The listing builds one solid part. Answer for the finished solid, in the listing's coordinates (mm). Round coordinates to 2 decimals unless told otherwise and drop trailing zeros. Write each loop counter-clockwise with the first axis right and the second up, starting at its lowest first coordinate (ties: lowest second). Pieces come first, ordered by that corner, then holes. Notation, with made-up numbers: (36.5, -28.5) -> (88.5, -28.5) arc R19 cw to (88.5, -13.5) -> close; hole circle Ø11 at (72.5, 80.5). An arc over 180 degrees is marked (long way). Write each question's results on one line, items separated by ' | '. Start each with the question number.
```python
from build123d import *

# Parameters (mm, degrees)
BOSS_EXTRUDE1_DEPTH = 692.15
CUT_EXTRUDE1_DEPTH  = 695.802886166


with BuildPart() as part:
    # Sketch1 → Boss-Extrude1 (new body)
    with BuildSketch(Plane.XY):
        Polygon((0, 0), (0, 60.325), (3.175, 60.325), (3.175, 57.15), (6.35, 57.15), (6.35, 6.35), (3.175, 6.35), (3.175, 0), align=None)
    extrude(amount=BOSS_EXTRUDE1_DEPTH)

    # Sketch2 → Cut-Extrude1 (cut, through all)
    with BuildSketch(Plane(origin=(0, 60.325, 0), x_dir=(1, 0, 0), z_dir=(0, 1, 0))):
        Polygon((0, 0), (6.35, -6.35), (6.35, 0), align=None)
    cut_extrude1 = extrude(amount=-CUT_EXTRUDE1_DEPTH, mode=Mode.SUBTRACT)

    # Mirror1: Cut-Extrude1 across plane
    add(cut_extrude1.mirror(Plane.XY.offset(346.075)), mode=Mode.SUBTRACT)


solid = part.part
```
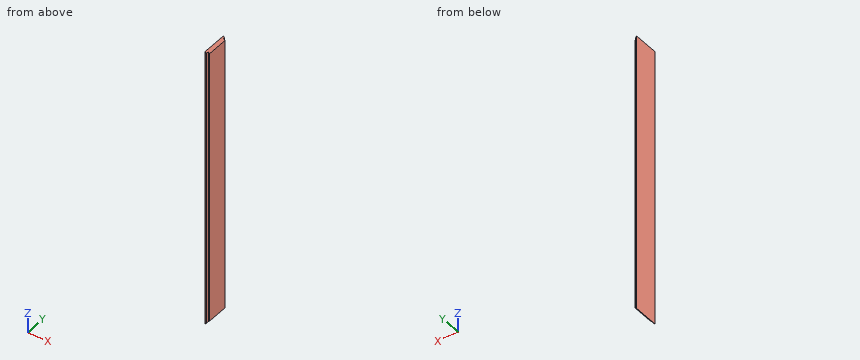
Q1. The part is cut by section A-A, the plane z = 43.5. Write down the section's boundary in (x, y) (3 decimals).
Q2. Each of these flat-tipped pins is pushed along its axis until it touches: pin 1 (2 mm diameter, centred on x = 5.5, y = 40, fed in from +Z); pin 2 (1 mm diameter, centred on x = 5, z = 195.5, fed in from -Y); pin 3 (3 mm diameter, centred on x = 4.5, y = 52, fed in from +Z). Where does it stop, or does it pass through?
Q3. Find the intervals of material crossed by line 1 (X direction, y = 5.5, z = 339.5) (3 decimals); line 2 (Y direction, x = 5, z = 587.5); line 3 (Z direction, x = 6.25, y = 46.5), in increasing order.
Answers follow:
1) outline: (0, 0) -> (3.175, 0) -> (3.175, 6.35) -> (6.35, 6.35) -> (6.35, 57.15) -> (3.175, 57.15) -> (3.175, 60.325) -> (0, 60.325) -> close
2) pin 1: z = 687.65 | pin 2: y = 6.35 | pin 3: z = 689.15
3) line 1: 0 to 3.175 | line 2: 6.35 to 57.15 | line 3: 6.25 to 685.9
